The listing builds one solid part. Answer for the finished solid, in the listing's coordinates (mm). Face numbers are marked on the shaded views. A direction names the side the tool comes from. Round coordinates to 2 decimals unless told otherwise and drop trailing zeros. Order: outer loops, then holes, each group sorted by start corner. A loop starts at its lowest first (then second) coordinate and runs counter-clockwise, first axis right, second up. Notation, with made-up numbers: (26, -6.5) - (67, -6.5) arc R23 ccw to (67, 30.5) - close; hole circle Ø11 at (-36, 16.25). An arc over 180 degrees is marked (long way). Write item = value, one per line.
from build123d import *

# Parameters (mm, degrees)
F0_W     = 125.545039773
F0_H     = 116.582095623
F1_DEPTH = 12.5
F2_R     = 5
F3_T     = -2.5


# Not quite as in the source:
# - a shell that OpenCascade refuses in one call is made with other operations: the cavity is built on its own and cut out


with BuildPart() as f1:
    # F0 (on Front) → F1 (new body, symmetric)
    with BuildSketch(Plane.XZ):
        Rectangle(F0_W, F0_H)
    extrude(amount=F1_DEPTH, both=True)

    # F2
    f2_edges = [f1.edges().sort_by_distance(p)[0] for p in [
        (62.77252, 0, 58.291048),
        (0, 12.5, 58.291048),
        (-62.77252, 0, 58.291048),
        (0, -12.5, 58.291048),
        (62.77252, 12.5, 0),
        (0, -12.5, -58.291048),
        (62.77252, -12.5, 0),
        (-62.77252, -12.5, 0),
        (-62.77252, 12.5, 0),
        (0, 12.5, -58.291048),
    ]]
    fillet(f2_edges, radius=F2_R)

    # F3: a shell. OpenCascade refuses it in one call, so the cavity is built on its own and cut out:
    # the body offset inwards by the wall thickness, plus a prism from it out through each open face.
    f3_core = offset(f1.part, amount=F3_T, mode=Mode.PRIVATE)
    f3_exits = [f3_core.faces().sort_by_distance(p)[0] for p in [
        (0, -10, 0),
    ]]
    add(f3_core, mode=Mode.SUBTRACT)
    extrude(f3_exits, amount=-F3_T, mode=Mode.SUBTRACT)


solid = f1.part
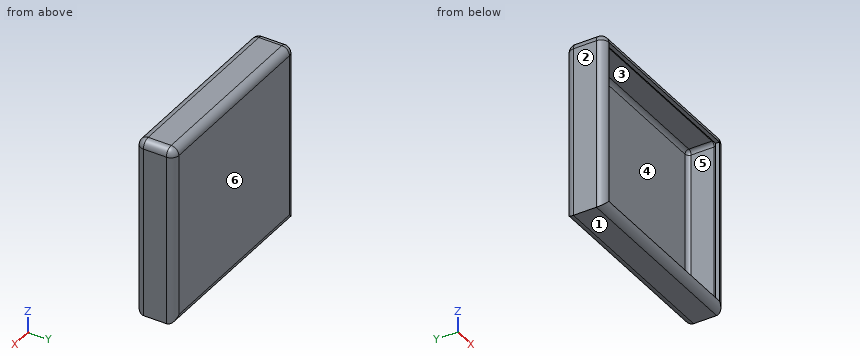
Q1. Section B-B on x = -12 is taken. Determine the outline of the cut face in (y, z).
Model answer:
outline = (-12.5, -53.29) arc R5 ccw to (-7.5, -58.29) - (7.5, -58.29) arc R5 ccw to (12.5, -53.29) - (12.5, 53.29) arc R5 ccw to (7.5, 58.29) - (-7.5, 58.29) arc R5 ccw to (-12.5, 53.29) - (-10, 53.29) arc R2.5 cw to (-7.5, 55.79) - (7.5, 55.79) arc R2.5 cw to (10, 53.29) - (10, -53.29) arc R2.5 cw to (7.5, -55.79) - (-7.5, -55.79) arc R2.5 cw to (-10, -53.29) - close
Q2. Find the intervals of material crossed by line 1 (Z direction, x = -15, y = -6); line 2 (X direction, y = 2.75, z = -28); line 3 (Y direction, x = -14.5, z = 33), in increasing order. Write a range as from..to.
Model answer:
line_1 = -58.29..-55.79, 55.79..58.29
line_2 = -62.77..-60.27, 60.27..62.77
line_3 = 10..12.5
Q3. Section C-C on z = -51 is taken. Determine the outline of the cut face in (x, y).
Model answer:
outline = (-62.77, -7.5) arc R5 ccw to (-57.77, -12.5) - (-57.77, -10) arc R2.5 cw to (-60.27, -7.5) - (-60.27, 7.5) arc R2.5 cw to (-57.77, 10) - (57.77, 10) arc R2.5 cw to (60.27, 7.5) - (60.27, -7.5) arc R2.5 cw to (57.77, -10) - (57.77, -12.5) arc R5 ccw to (62.77, -7.5) - (62.77, 7.5) arc R5 ccw to (57.77, 12.5) - (-57.77, 12.5) arc R5 ccw to (-62.77, 7.5) - close
Q4. For the marked faces 4, 5 and 6, determine the directions among +Z, -Z, +X, -X, +Y, -Y from which every point of the face is accessible in a straight line to the end or side of a thin tool.
Model answer:
face_4 = -Y
face_5 = none
face_6 = +Z, -Z, +X, -X, +Y
Q5. Section A-A on y = 0.25 is taken. Determine the outline of the cut face in (x, z).
Model answer:
outline = (-62.77, -58.29) - (62.77, -58.29) - (62.77, 53.29) arc R5 ccw to (57.77, 58.29) - (-57.77, 58.29) arc R5 ccw to (-62.77, 53.29) - close; hole (-60.27, -55.79) - (60.27, -55.79) - (60.27, 53.29) arc R2.5 ccw to (57.77, 55.79) - (-57.77, 55.79) arc R2.5 ccw to (-60.27, 53.29) - close
Q6. Flat-ended cylindrical pins translate along their axes: P1, Ø8, axis at y = 9.5, z = -32, coming from the +X side; P2, Ø3, axis at x = -3, y = -11.5, coming from the +Z side; P3, Ø3, axis at x = -11, z = -7, coming from the -Y side; P4, Ø0.8, axis at y = -12, z = -7.5, coming from the +X side. Find the tip coordinate at first contact, or state that the pin passes through.
Model answer:
P1 = 62.77
P2 = 57.62
P3 = 10
P4 = 60.63
Q7. Determine the mould class of the marked faces 1, 2 and 3 for opening direction Z: released by +Z, released by -Z, zero draft, split by the parting line, or undercut.
Model answer:
face_1 = released by -Z
face_2 = zero draft
face_3 = undercut
